Geometry check sheet. Reference: the model listing, model coordinates, mm. Face numbers are marked on the shaded views. A direction names the side the tool comes from. Round coordinates to 2 decimals unless told otherwise and drop trailing zeros. Order: outer loops, then holes, each group sorted by start corner. A loop starts at its lowest first (then second) coordinate and runs counter-clockwise, first axis right, second up. Notation, with made-up numbers: (-8.75, 7.25) - (19.25, 7.25) arc R11 ccw to (19.25, 15.25) - close; hole circle Ø2 at (89.5, -7.5). An arc over 180 degrees is marked (long way). Return JSON: item names as keys, results as strings. Group by question number.
Q1. Sectioned sample at A-A, the plane x = 0. Record the cut outline in (y, z).
Q2. Gauge pin test, flat ends, axial feed: pin 1 Ø5 at (x, z) = (0, 0) entering from +Y; pin 2 Ø7 at (x, z) = (0, 0) entering from +Y; pin 3 Ø4 at (y, z) = (12, 3.5) entering from +X. Record the tip position at first contact, or that the pin passes through.
Q3. Sectioned sample at C-C, the plane y = 14. Record the cut outline in (x, z), then the cut area to 3 significant figures.
Q4. Sectioned sample at D-D, the plane y = 8. Record the cut outline in (x, z), then the cut area to 3 significant figures.
Q5. Sectioned sample at B-B, the plane z = 0. Record the cut outline in (x, y).
Q6. Material ranges on line 1 along X through (y, z) = (22.5, 0); line 2 along X through (y, z) = (15.1, 0); line 3 along Z through (x, y) = (-3.5, 25.25), recorded low to high.
Q7. Tool access check on the marked faces 1 and 2. Record the directions out of +Z, -Z, +X, -X, +Y, -Y that give a thin tool (end or side, any length) a straight path to the whole face; none if there is none.
Q8. Draft check along Z on the marked faces 3, 4 and 5. Enter one of: pulls with the +Z half, pulls with the -Z half, needs draft (parallel to the pull), parting line crosses it, or undercut.
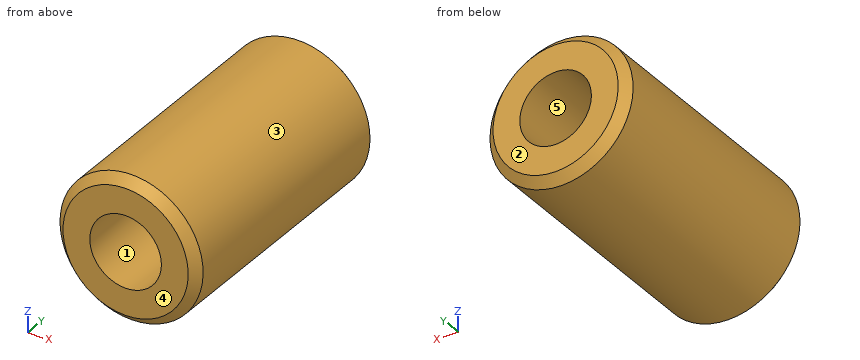
```python
from build123d import *

# Parameters (mm, degrees)
CHAMFER_1_SIZE = 1


with BuildPart() as part:
    # Эскиз1 → Повернуть1 (revolve)
    with BuildSketch(Plane.XY, mode=Mode.PRIVATE) as revolve_1_sk:
        Polygon((8, 0), (8, 30), (4, 30), (4, 20), (1, 17), (1, 13), (4, 10), (4, 0), align=None)
    revolve(revolve_1_sk.sketch.rotate(Axis((0, 0, 0), (0, 1, 0)), 90), axis=Axis((0, 0, 0), (0, 1, 0)))

    # Фаска1
    chamfer_1_edges = [part.edges().sort_by_distance(p)[0] for p in [
        (0, 0, 8),
        (0, 30, 8),
    ]]
    chamfer(chamfer_1_edges, length=CHAMFER_1_SIZE)


solid = part.part
```
Reply:
{
 "1": {"outline": "(0, -7) - (1, -8) - (29, -8) - (30, -7) - (30, -4) - (20, -4) - (17, -1) - (13, -1) - (10, -4) - (0, -4) - close; (0, 4) - (10, 4) - (13, 1) - (17, 1) - (20, 4) - (30, 4) - (30, 7) - (29, 8) - (1, 8) - (0, 7) - close"},
 "2": {"pin 1": "y = 18.5", "pin 2": "y = 19.5", "pin 3": "x = 7.86"},
 "3": {"outline": "circle Ø16 at (0, 0); hole circle Ø2 at (0, 0)", "area": "198 mm^2"},
 "4": {"outline": "circle Ø16 at (0, 0); hole circle Ø8 at (0, 0)", "area": "151 mm^2"},
 "5": {"outline": "(-8, 1) - (-7, 0) - (-4, 0) - (-4, 10) - (-1, 13) - (-1, 17) - (-4, 20) - (-4, 30) - (-7, 30) - (-8, 29) - close; (1, 13) - (4, 10) - (4, 0) - (7, 0) - (8, 1) - (8, 29) - (7, 30) - (4, 30) - (4, 20) - (1, 17) - close"},
 "6": {"line 1": "-8 to -4, 4 to 8", "line 2": "-8 to -1, 1 to 8", "line 3": "-7.19 to -1.94, 1.94 to 7.19"},
 "7": {"face 1": "-Y", "face 2": "+Z, -Z, +X, -X, +Y"},
 "8": {"face 3": "parting line crosses it", "face 4": "needs draft", "face 5": "undercut"}
}
